Autodesk Inventor part; units mm, degrees
ref_plane "YZ Plane" through (0, 0, 0) normal (1, 0, 0) x (0, 1, 0)
ref_plane "XZ Plane" through (0, 0, 0) normal (0, 1, 0) x (-1, 0, 0)
ref_plane "XY Plane" through (0, 0, 0) normal (0, 0, 1) x (1, 0, 0)
sketch "草圖1" plane through (0, 0, 0) normal (0, 0, 1) x (1, 0, 0)
  circle A0 centre (0, 0) radius 30
  circle A1 centre (0, 0) radius 15
  dimension "d0" = 60
  dimension "d1" = 30
extrude "擠出1" add sketch "草圖1" along normal blind 7.5
sketch "草圖2" plane through (0, 0, 0) normal (0, 0, -1) x (-1, 0, 0)
  circle A0 centre (0, 0) radius 20
  circle A1 centre (0, 0) radius 34.9484
  dimension "d4" = 40
extrude "擠出2" cut sketch "草圖2" against normal blind 0.5
sketch "草圖3" plane through (0, 0, 7.5) normal (0, 0, 1) x (1, 0, 0)
  circle A0 centre (0, 0) radius 19
  circle A1 centre (0, 0) radius 30.8877
  dimension "d7" = 38
extrude "擠出3" cut sketch "草圖3" against normal blind 3
chamfer "倒角1" distance 3 angle 45 1 edges at (-30, 0, 4.5)
chamfer "倒角2" distance 0.3 angle 45 2 edges at (-15, 0, 7.5) (-19, 0, 7.5)
chamfer "倒角3" distance 0.3 angle 45 1 edges at (-15, 0, 0)
properties part number "KMB601機械油封墊片(T=7.5-外徑60)"
Could you check a few things on this model? Use its own coordinates, in mm. A direction names the side the tool comes from. Coordinates: 2 decimals unless noted, no trailing zeros. Write each loop counter-clockwise with the first axis right and the second up, starting at its lowest first coordinate (ties: lowest second). Pieces come first, ordered by that corner, then holes. Notation, with made-up numbers: (-5.75, 15.25) - (19.25, 15.25) arc R22 ccw to (19.25, 31.25) - close; hole circle Ø7 at (67, 78.25). An arc over 180 degrees is marked (long way). Write item = value, one per line.
1) Will these pins go through, and if not, where does the flat tip stop? pin 1 Ø2 at (y, z) = (5, 4) entering from -X; pin 2 Ø3 at (x, z) = (21.5, 2.5) entering from -Y; pin 3 Ø3 at (x, z) = (21, 1) entering from +Y.
Result set:
pin_1 = -28.07
pin_2 = -22.01
pin_3 = 22.8
2) Suppose I cut it at A-A on y = 0. Please give me the cut outline in (x, z), plus the area to 3 significant figures.
Result set:
outline = (-30, 0.5) - (-20, 0.5) - (-20, 0) - (-15.3, 0) - (-15, 0.3) - (-15, 7.2) - (-15.3, 7.5) - (-18.7, 7.5) - (-19, 7.2) - (-19, 4.5) - (-27, 4.5) - (-30, 1.5) - close; (15, 0.3) - (15.3, 0) - (20, 0) - (20, 0.5) - (30, 0.5) - (30, 1.5) - (27, 4.5) - (19, 4.5) - (19, 7.2) - (18.7, 7.5) - (15.3, 7.5) - (15, 7.2) - close
area = 140 mm2
3) Suppose I cut it at C-C on z = 2.5. Please give me the cut outline in (x, y).
Result set:
outline = circle Ø58 at (0, 0); hole circle Ø30 at (0, 0)
4) For faces 4 (the flat face through (-6, -20, 0.5)), 5 (the cylindrical face through (8.767, -16.856, 5.869)), 6 (the flat face through (-7, -14, 7.5)), which set-ups out of +Z, -Z, +X, -X, +Y, -Y let a thin tool reach every point of the face, with its end or its side?
Result set:
face_4 = -Z
face_5 = +Z
face_6 = +Z, +X, -X, +Y, -Y
5) Please list where these lines run through material, in increasing order: line 1 (Y direction, x = 0, z = 5); line 2 (Z direction, x = -19, y = 3); line 3 (Y direction, x = 1.5, z = 1.75). Write a range as [from, to].
Result set:
line_1 = [-19, -15], [15, 19]
line_2 = [0, 4.5]
line_3 = [-29.71, -14.92], [14.92, 29.71]
6) We'd pull the mould along Y, two halves only. Please class faces 1 (the cylindrical face through (-14.985, -0.66, 3.702)), 2 (the cylindrical face through (-29.97, -1.32, 0.99)), 3 (the flat face through (-5, -15, 0)): +Y half, -Y half, draft (parallel to the pull), parting line (faces both ways), or undercut.
Result set:
face_1 = undercut
face_2 = parting line
face_3 = draft
